from build123d import *

# Parameters (mm, degrees)
SM_BASE_FLANGE_1_DEPTH = 100
SKETCH_3_W             = 60
SKETCH_3_H             = 50
CUT_EXTRUDE_1_DEPTH    = 120.933314805
SKETCH_4_R             = 15
CUT_EXTRUDE_2_DEPTH    = 120.268604419
SKETCH_5_R             = 3
CUT_EXTRUDE_3_DEPTH    = 120.268604419
FILLET_1_R             = 10
CUT_EXTRUDE_4_DEPTH    = 120.268604419


# Sheet-metal steps are written as plain solids
with BuildPart() as part:
    # Sketch 1 → 基体-法兰1 (new body)
    with BuildSketch(Plane.XY):
        with BuildLine():
            Line((0, 25), (0, 0.7366))
            ThreePointArc((0, 0.7366), (0.215745145, 0.215745145), (0.7366, 0))
            Line((0.7366, 0), (60, 0))
            Line((60, 0), (60, -3))
            Line((60, -3), (0.7366, -3))
            ThreePointArc((0.7366, -3), (-1.905575199, -1.905575199), (-3, 0.7366))
            Line((-3, 0.7366), (-3, 25))
            Line((-3, 25), (0, 25))
        make_face()
    extrude(amount=-SM_BASE_FLANGE_1_DEPTH)

    # 草图3 → 切除-拉伸1 (cut, through all)
    with BuildSketch(Plane(origin=(0, 25, 0), x_dir=(1, 0, 0), z_dir=(0, 1, 0))):
        with Locations((30, 75)):
            Rectangle(SKETCH_3_W, SKETCH_3_H)
    extrude(amount=-CUT_EXTRUDE_1_DEPTH, mode=Mode.SUBTRACT)

    # 草图4 → 切除-拉伸2 (cut, through all)
    with BuildSketch(Plane(origin=(0, 0, 0), x_dir=(1, 0, 0), z_dir=(0, 1, 0))):
        with Locations(Location((35, 25, 0), (0, 0, 270))):
            Circle(SKETCH_4_R)
    extrude(amount=-CUT_EXTRUDE_2_DEPTH, mode=Mode.SUBTRACT)

    # 草图5 → 切除-拉伸3 (cut, through all)
    with BuildSketch(Plane(origin=(0, 0, 0), x_dir=(0, 0, -1), z_dir=(1, 0, 0))):
        with Locations(Location((75, 12.8683, 0), (0, 0, 90))):
            Circle(SKETCH_5_R)
        with Locations(Location((90, 12.8683, 0), (0, 0, 90))):
            Circle(SKETCH_5_R)
    extrude(amount=-CUT_EXTRUDE_3_DEPTH, mode=Mode.SUBTRACT)

    # 圆角1
    fillet_1_edges = [part.edges().sort_by_distance(p)[0] for p in [
        (60, -1.5, -50),
        (-1.5, 25, 0),
        (60, -1.5, 0),
    ]]
    fillet(fillet_1_edges, radius=FILLET_1_R)

    # 草图6 → 切除-拉伸4 (cut, through all)
    with BuildSketch(Plane(origin=(0, 0, 0), x_dir=(0, 0, -1), z_dir=(1, 0, 0))):
        Polygon((100, 25), (95, 25), (100, 20), align=None)
        Polygon((100, 2.073322779), (100, -2.926677221), (95, -2.926677221), align=None)
    extrude(amount=-CUT_EXTRUDE_4_DEPTH, mode=Mode.SUBTRACT)


solid = part.part
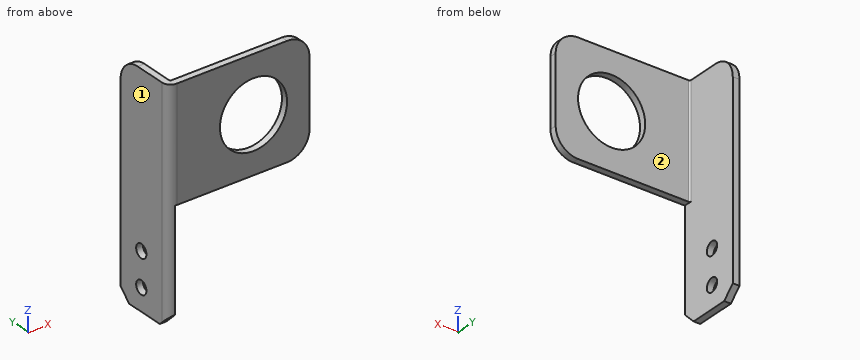
Here's how the part is built. I have some questions about the finished solid (model axes, mm). Face numbers are marked on the shaded views. A direction names the side the tool comes from. Coordinates: 2 decimals unless noted, no trailing zeros. Order: outer loops, then holes, each group sorted by start corner. A loop starts at its lowest first (then second) coordinate and runs counter-clockwise, first axis right, second up. Notation, with made-up numbers: (44, 41.5) -> (57, 41.5) arc R18 cw to (57, 60.5) -> close; hole circle Ø2 at (27, -2). An arc over 180 degrees is marked (long way). Answer in a Markdown table with one row per item.
(1) I want a section at B-B on z = -25. List the corners of the cut face in (x, y) for me.
Answer key:
| item | result |
|---|---|
| outline | (-3, 0.74) arc R3.74 ccw to (0.74, -3) -> (20, -3) -> (20, 0) -> (0.74, 0) arc R0.74 cw to (0, 0.74) -> (0, 25) -> (-3, 25) -> close; (50, -3) -> (60, -3) -> (60, 0) -> (50, 0) -> close |
(2) Please list where this line runs through material, in increasing order: probe 1 along Y at (x, z) = (10.5, -10).
Answer key:
| item | result |
|---|---|
| probe 1 | -3 to 0 |
(3) I want a section at C-C on z = -90. List the corners of the cut face in (x, y) for me, then the cut area to 3 significant figures.
Answer key:
| item | result |
|---|---|
| outline | (-3, 0.74) arc R3.74 ccw to (0, -2.93) -> (0, 9.87) -> (-3, 9.87) -> close; (-3, 15.87) -> (0, 15.87) -> (0, 25) -> (-3, 25) -> close |
| area | 63.0 mm^2 |
(4) Will these pins go through, and if not, where does the flat tip stop? pin 1 Ø8.5 at (y, z) = (8.5, -70.5) entering from +X; pin 2 Ø5.5 at (y, z) = (12.87, -75) entering from +X; pin 3 Ø3 at (x, y) = (22.5, -1) entering from -Z; pin 4 Ø3 at (x, z) = (20, -35) entering from +Y.
Answer key:
| item | result |
|---|---|
| pin 1 | x = 0 |
| pin 2 | through |
| pin 3 | z = -50 |
| pin 4 | y = 0 |
(5) On a 3-axis mill with a long thin cutter (end or side, diameter ignored), from which of +Z, -Z, +X, -X, +Y, -Y can I reach the whole of each face in a straight line? I mean the marked faces 1 and 2. Say none if no direction works.
Answer key:
| item | result |
|---|---|
| face 1 | +Z, -Z, -X, +Y, -Y |
| face 2 | +Z, -Z, +X, +Y |
(6) I want a section at A-A on x = 35. List the corners of the cut face in (y, z) for me, then the cut area to 3 significant figures.
Answer key:
| item | result |
|---|---|
| outline | (-3, -50) -> (0, -50) -> (0, -40) -> (-3, -40) -> close; (-3, -10) -> (0, -10) -> (0, 0) -> (-3, 0) -> close |
| area | 60.0 mm^2 |
(7) I want a section at D-D on y = 6.5. List the corners of the cut face in (x, z) for me.
Answer key:
| item | result |
|---|---|
| outline | (-3, -100) -> (0, -100) -> (0, 0) -> (-3, 0) -> close |
